Could you check a few things on this model? Use its own coordinates, in mm. Give positions to 0.01 mm unless a question says otherwise; leave off trailing zeros. Order: outer loops, then holes, each group sorted by start corner. A loop starts at its lowest first (then second) coordinate and runs counter-clockwise, first axis right, second up. Notation, with made-up numbers: (38.25, -19.5) - (82.25, -19.5) arc R20 cw to (82.25, -12.5) - close; hole circle Ø2 at (-22, 50). An arc over 180 degrees is marked (long way). Put each result on its own line as item: value.
Autodesk Inventor part; units mm, degrees
ref_plane "YZ Plane" through (0, 0, 0) normal (1, 0, 0) x (0, 1, 0)
ref_plane "XZ Plane" through (0, 0, 0) normal (0, 1, 0) x (-1, 0, 0)
ref_plane "XY Plane" through (0, 0, 0) normal (0, 0, 1) x (1, 0, 0)
sketch "Sketch1" plane through (0, 0, 0) normal (0, 0, 1) x (1, 0, 0)
  circle A0 centre (0, 0) radius 1.675
  circle A1 centre (25, 0) radius 1.675
  line L0 (0, 0) -> (0, 1.675)
  circle A2 centre (0, 125) radius 1.675
  circle A3 centre (25, 125) radius 1.675
  line L1 (33, -8) -> (-57.1446, -8)
  line L2 (-57.1446, -8) -> (-57.1446, 137.5528)
  line L3 (-57.1446, 137.5528) -> (33, 137.5528)
  line L4 (33, 137.5528) -> (33, -8)
  line L5 (-57.1446, 64.7764) -> (33, 64.7764)
  circle A4 centre (-42.1446, 64.7764) radius 9.5
  point P0 (0, 126.675)
  dimension "d0" = 3.35
  dimension "d1" = 3.35
  dimension "d2" = 25
  dimension "d5" = 125
  dimension "d10" = 8
  dimension "d11" = 8
  dimension "d12" = 12.5528
  dimension "d13" = 19
  dimension "d14" = 15
extrude "Plate1" add sketch "Sketch1" along normal blind 1.5 contours L1 L2 L5 A4 L4 | L5 A4 L2 L3 L4
chamfer "Corner Chamfer1" distance 40 distance2 65 1 edges at (-57.1446, 137.5528, 0.75) measured on face at (2.9518, 137.5528, 0.5)
chamfer "Corner Chamfer2" distance 40 distance2 65 1 edges at (-57.1446, -8, 0.75) measured on face at (-27.0964, -8, 0.5)
fillet "Corner Round1" radius 12 2 edges at (-57.1446, 72.5528, 0.75) (-57.1446, 57, 0.75)
chamfer "Corner Chamfer3" distance 6 angle 45 4 edges at (33, 137.5528, 0.75) (-17.1446, 137.5528, 0.75) (-17.1446, -8, 0.75) (33, -8, 0.75)
equation "\"d0\" = rivet_diameter"
equation "\"d1\" = rivet_diameter"
equation "\"d15\" = Thickness"
equation "\"Thickness\" = plate_thickness"
equation "\"BendRadius\" = Thickness"
equation "\"BendReliefWidth\" = Thickness"
equation "\"BendReliefDepth\" = 0.5 * Thickness"
equation "\"CornerReliefSize\" = 4 * Thickness"
equation "\"MinimumRemnant\" = 2 * Thickness"
equation "\"TransitionRadius\" = BendRadius"
equation "\"JacobiRadiusSize\" = BendRadius"
equation "\"GapSize\" = Thickness"
equation "\"A_joint_diameter\" = 16"
equation "\"A_B_spacing\" = 2"
equation "\"A_joint_tolerance\" = 3"
equation "\"l___________\" = 0"
equation "\"l__________\" = 0"
equation "\"l_________\" = 0"
equation "\"rivet_diameter\" = 3.35"
equation "\"plate_thickness\" = 1.5"
equation "\"l________\" = 0"
equation "\"L_Piston_Top\" = 25"
equation "\"L_Piston_Bottom\" = 21"
properties part number "Piston_A_beam_hinge"
1) Suppose I cut it at C-C, the plane x = -38. List the corners of the cut face in (y, z) for me.
Filled in:
outline: (25.89, 0) - (56.23, 0) - (56.23, 1.5) - (25.89, 1.5) - close; (73.32, 0) - (103.66, 0) - (103.66, 1.5) - (73.32, 1.5) - close
2) If I drill on line 1 (Y direction, x = 25, z = 0.65) (3 decimals); line 2 (X direction, y = 125, z = 0.7) (3 decimals); line 3 (X direction, y = 62, z = 1.2), over which ranges is the centre line in solid material (lowest first)? Write a range as [from, to].
Filled in:
line 1: y = [-8, -1.675], [1.675, 123.325], [126.675, 137.553]
line 2: x = [-24.869, -1.675], [1.675, 23.325], [26.675, 33]
line 3: x = [-57.14, -51.23], [-33.06, 33]
3) We'd pull the mould along X, two halves only. Please class faces 1 (the flat face through (30, -5, 1)), 2 (the flat face through (-3, 66, 1.5)), 3 (the cylindrical face through (-0.22, 123.34, 0.74)): pulls with the +X half, pulls with the -X half, needs draft (parallel to the pull), parting line crosses it, or undercut.
Filled in:
face 1: pulls with the +X half
face 2: needs draft
face 3: undercut
4) Suppose I cut it at A-A, the plane x = 0. List the corners of the cut face in (y, z) for me (3 decimals).
Filled in:
outline: (-8, 0) - (-1.675, 0) - (-1.675, 1.5) - (-8, 1.5) - close; (1.675, 0) - (123.325, 0) - (123.325, 1.5) - (1.675, 1.5) - close; (126.675, 0) - (137.553, 0) - (137.553, 1.5) - (126.675, 1.5) - close
5) Suppose I cut it at B-B, the plane y = 0. List the corners of the cut face in (x, z) for me (3 decimals).
Filled in:
outline: (-22.068, 0) - (-1.675, 0) - (-1.675, 1.5) - (-22.068, 1.5) - close; (1.675, 0) - (23.325, 0) - (23.325, 1.5) - (1.675, 1.5) - close; (26.675, 0) - (33, 0) - (33, 1.5) - (26.675, 1.5) - close
6) I'm going to push a flat-ended pin straight in: pin 1 (3 mm diameter, centred on x = 0, y = 0, fed in from +Z). Where does the tip first touch, or does it pass through?
Filled in:
pin 1: passes through
7) Suppose I cut it at D-D, the plane y = 98. List the corners of the cut face in (x, z) for me.
Filled in:
outline: (-41.48, 0) - (33, 0) - (33, 1.5) - (-41.48, 1.5) - close
